Geometry check sheet. Reference: the model listing, model coordinates, mm. Face numbers are marked on the shaded views. A direction names the side the tool comes from. Round coordinates to 2 decimals unless told otherwise and drop trailing zeros. Loops run counter-clockwise (first coordinate to the right, second up) from the corner with the lowest first, then second, coordinate; pieces in that order, holes last. Notation, with made-up numbers: M -10.5,11 L 14.5,11 A7 cw 14.5,23 Z; hole C 61,49 d8. An arc over 180 degrees is marked long. Use one line per item in the form item = value. Start each with the question number.
1. Draft check along Y on the marked faces 3, 4 and 5. Enter one of: pulls with the +Y half, pulls with the -Y half, needs draft (parallel to the pull), parting line crosses it, or undercut.
2. Cross-section at A-A (y = 0). Record the boundary of the cut face in (x, z).
3. Material ranges on line 1 (Y direction, x = 0, z = 12.25); line 2 (Z direction, x = 2.5, y = -4); line 3 (Y direction, x = -2.5, z = 12), recorded low to high.
4. Cross-section at C-C (z = 13.5). Record the boundary of the cut face in (x, y), then the cut area to 3 significant figures.
5. Set-up check for the marked faces 1 and 2: record each of +Z, -Z, +X, -X, +Y, -Y from which the full face is reachable in a straight line by a thin tool's end or side.
6. Go/stop test with flat-tipped pins: pin 1 (5 mm diameter, centred on x = 0.5, y = -3, fed in from -Z); pin 2 (4 mm diameter, centred on y = -4, z = 11, fed in from +X); pin 3 (3 mm diameter, centred on y = 1, z = 14, fed in from +X). Record where each tip stops, or that it passes through.
7. Cross-section at D-D (x = 3.75). Record the boundary of the cut face in (y, z), then the cut area to 3 significant figures.
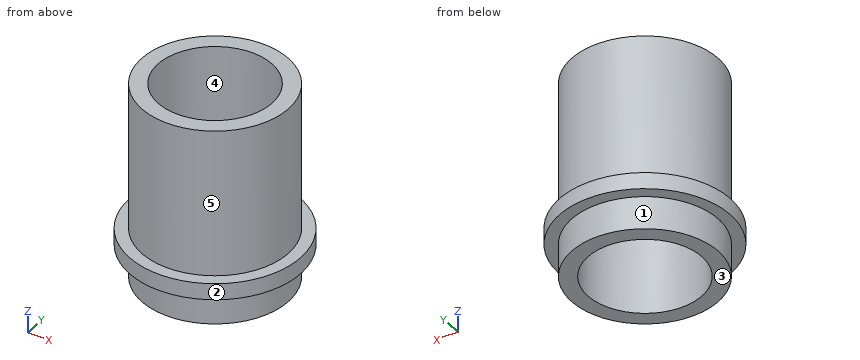
```python
from build123d import *

# Parameters (mm, degrees)
BOSS_EXTRUDE1_START = 8
SKETCH1_R           = 4.5
SKETCH1_R_2         = 3.5
BOSS_EXTRUDE1_DEPTH = 12
BOSS_EXTRUDE2_START = -2
SKETCH2_R           = 5.25
SKETCH2_R_2         = 3.5
BOSS_EXTRUDE2_DEPTH = 1


with BuildPart() as part:
    # Sketch1 → Boss-Extrude1 (new body)
    with BuildSketch(Plane.XY.offset(BOSS_EXTRUDE1_START)):
        Circle(SKETCH1_R)
        Circle(SKETCH1_R_2, mode=Mode.SUBTRACT)
    extrude(amount=BOSS_EXTRUDE1_DEPTH)

    # Sketch2 → Boss-Extrude2 (add)
    with BuildSketch(Plane(origin=(0, 0, 8), x_dir=(-1, 0, 0), z_dir=(0, 0, -1)).offset(BOSS_EXTRUDE2_START)):
        Circle(SKETCH2_R)
        Circle(SKETCH2_R_2, mode=Mode.SUBTRACT)
    extrude(amount=-BOSS_EXTRUDE2_DEPTH)


solid = part.part
```
Reported:
q1.face_3 = needs draft
q1.face_4 = undercut
q1.face_5 = parting line crosses it
q2.outline = M -5.25,10 L -4.5,10 L -4.5,8 L -3.5,8 L -3.5,20 L -4.5,20 L -4.5,11 L -5.25,11 Z; M 3.5,8 L 4.5,8 L 4.5,10 L 5.25,10 L 5.25,11 L 4.5,11 L 4.5,20 L 3.5,20 Z
q3.line_1 = -4.5 to -3.5, 3.5 to 4.5
q3.line_2 = 10 to 11
q3.line_3 = -3.74 to -2.45, 2.45 to 3.74
q4.outline = C 0,0 d9; hole C 0,0 d7
q4.area = 25.1 mm²
q5.face_1 = -Z
q5.face_2 = +Z, -Z
q6.pin_1 = 8
q6.pin_2 = 4.85
q6.pin_3 = 4.5
q7.outline = M -3.67,10 L -2.49,10 L -2.49,8 L 2.49,8 L 2.49,10 L 3.67,10 L 3.67,11 L 2.49,11 L 2.49,20 L -2.49,20 L -2.49,11 L -3.67,11 Z
q7.area = 62.1 mm²
